Solid Edge part; units mm, degrees
sketch "Sketch1" plane through (0, 0, 0) normal (0, 0, 1) x (1, 0, 0)
  line L0 (0, 0) -> (0, 12.7)
  line L1 (0, 12.7) -> (50.8, 12.7)
  line L2 (50.8, 12.7) -> (50.8, 0)
  line L3 (50.8, 0) -> (0, 0)
  dimension "D1" = 50.8
extrude "Protrusion1" add sketch "Sketch1" along normal blind 1.016
sketch "Sketch2" plane through (50.8, 9.525, 0.381) normal (1, 0, 0) x (0, 1, 0)
  circle A0 centre (3.175, 1.778) radius 2.159
  dimension "D1" = 3.175
extrude "ExtrudedProtrusion_2" add sketch "Sketch2" against normal blind 50.8
hole "Hole_1" at (44.45, 4.7625, 1.016) direction (0, 0, -1) diameter 3.175 end up to next
hole "Hole1" at (6.35, 4.7625, 1.016) direction (0, 0, -1) diameter 3.175 end up to next
properties part number "HARDWARE" material "Steel"
Design review of the part built by this model. Coordinates are the model's own, in mm. Round coordinates to 2 decimals unless told otherwise and drop trailing zeros. Write each loop counter-clockwise with the first axis right and the second up, starting at its lowest first coordinate (ties: lowest second). Pieces come first, ordered by that corner, then holes. Notation, with made-up numbers: (46, -24) -> (99, -24) arc R23 cw to (99, -5) -> close; hole circle Ø2 at (73.5, 20). An arc over 180 degrees is marked (long way). Answer in a Markdown table with one row per item.
Q1. Clearance check with flat-ended pins moving along their axes: pin 1 Ø6 at (x, y) = (39, 10) entering from +Z; pin 2 Ø3.5 at (x, y) = (44.45, 4.76) entering from +Z; pin 3 Ø1.5 at (y, z) = (4.5, 2.5) entering from +X (1 decimal). State where each tip first meets the part, or that it passes through.
The answers:
| item | result |
|---|---|
| pin 1 | z = 4.32 |
| pin 2 | z = 1.02 |
| pin 3 | through |
Q2. Take a section at A-A, the plane x = 44.45. State the section outline as (y, z) points (3 decimals).
The answers:
| item | result |
|---|---|
| outline | (0, 0) -> (3.175, 0) -> (3.175, 1.016) -> (0, 1.016) -> close; (6.35, 0) -> (12.7, 0) arc R2.159 ccw (long way) to (10.868, 1.016) -> (6.35, 1.016) -> close |
Q3. Take a section at C-C, the plane y = 10. State the section outline as (x, z) points, then the cut area to 3 significant figures.
The answers:
| item | result |
|---|---|
| outline | (0, 0) -> (50.8, 0) -> (50.8, 1.02) -> (0, 1.02) -> close |
| area | 51.6 mm² |
Q4. Draft analysis for pull direction X (two halves, no side actions). For faces 1 (the face through (0, 11, 2)), 2 (the face through (26, 6, 0)), 3 (the face through (42.9, 5.1, 0.5)), 4 (the face through (5.38, 6.02, 0.52)), state which applies: +X half, -X half, draft (parallel to the pull), parting line (faces both ways), or undercut.
The answers:
| item | result |
|---|---|
| face 1 | -X half |
| face 2 | draft |
| face 3 | undercut |
| face 4 | undercut |
Q5. To check wall thickness, follow L1, parallel to Z at x = 12.5, y = 0.5; L2, parallel to X at y = 4.5, z = 0.35; L3, parallel to Y at x = 44.45, z = 0.3 (3 decimals). State the ranges of each line that lie inside material, in increasing order. Write a range as [from, to].
The answers:
| item | result |
|---|---|
| L1 | [0, 1.02] |
| L2 | [0, 4.78], [7.92, 42.88], [46.02, 50.8] |
| L3 | [0, 3.175], [6.35, 13.798] |
Q6. Take a section at D-D, the plane x = 20. State the section outline as (y, z) points.
The answers:
| item | result |
|---|---|
| outline | (0, 0) -> (12.7, 0) arc R2.16 ccw (long way) to (10.87, 1.02) -> (0, 1.02) -> close |
Q7. Take a section at B-B, the plane z = 0.5. Count the separate pieces of the cut face and the enclosed holes in it, then the cut area to 3 significant figures.
The answers:
| item | result |
|---|---|
| separate pieces | 1 |
| enclosed holes | 2 |
| area | 700 mm² |
